Could you check a few things on this model? Use its own coordinates, in mm. A direction names the side the tool comes from. Round coordinates to 2 decimals unless told otherwise and drop trailing zeros. Loops run counter-clockwise (first coordinate to the right, second up) from the corner with the lowest first, then second, coordinate; pieces in that order, holes last. Notation, with made-up numbers: (35.5, -36.75) -> (77.5, -36.75) arc R36 cw to (77.5, -0.75) -> close; hole circle Ø6 at (47, 64). An arc over 180 degrees is marked (long way). One line per item, written item: value.
Autodesk Inventor part; units mm, degrees
ref_plane "YZ Plane" through (0, 0, 0) normal (1, 0, 0) x (0, 1, 0)
ref_plane "XZ Plane" through (0, 0, 0) normal (0, 1, 0) x (-1, 0, 0)
ref_plane "XY Plane" through (0, 0, 0) normal (0, 0, 1) x (1, 0, 0)
sketch "Boceto1" plane through (0, 0, 0) normal (0, 0, 1) x (1, 0, 0)
  point P0 (0, 0)
sketch "Boceto2" plane through (0, 0, 0) normal (0, 0, 1) x (1, 0, 0)
  line L0 (0, 0) -> (0, 200)
  line L1 (0, 200) -> (600, 200)
  line L2 (600, 200) -> (600, 0)
  line L3 (600, 0) -> (0, 0)
  dimension "d0" = 200
  dimension "d1" = 600
  dimension "d2" = 200
  dimension "d3" = 600
extrude "Extrusión1" add sketch "Boceto2" along normal blind 300
shell "Vaciado1" thickness 10 removed faces 1 at (400, 0, 100)
sketch "Boceto3" plane through (0, 200, 0) normal (0, 1, 0) x (1, 0, 0)
  point P0 (0, 0)
sketch "Boceto4" plane through (0, 200, 0) normal (0, 1, 0) x (1, 0, 0)
  point P0 (0, 0)
sketch "Boceto5" plane through (0, 200, 0) normal (0, 1, 0) x (1, 0, 0)
  point P0 (0, 0)
sketch "Boceto6" plane through (0, 200, 0) normal (0, 1, 0) x (1, 0, 0)
  circle A0 centre (300, -150) radius 15
  point P0 (0, 0)
  dimension "d9" = 30
extrude "Extrusión2" cut sketch "Boceto6" against normal blind 33.25
sketch "Boceto7" plane through (0, 200, 0) normal (0, 1, 0) x (1, 0, 0)
  point P0 (0, 0)
sketch "Boceto8" plane through (600, 0, 0) normal (1, 0, 0) x (0, 0, -1)
  circle A0 centre (-22.0681, 21.036) radius 17.5
  circle A1 centre (-69.9749, 21.036) radius 17.5
  point P0 (0, 0)
  dimension "d12" = 35
  dimension "d13" = 35
extrude "Extrusión3" cut sketch "Boceto8" against normal blind 33.25
sketch "Boceto9" plane through (0, 0, 0) normal (-1, 0, 0) x (0, 0, 1)
  arc A0 (10, 8.3628) -> (10, 33.7092) centre (22.0681, 21.036) ccw
  circle A1 centre (22.0681, 21.036) radius 17.5
  circle A2 centre (66.1324, 21.036) radius 17.5
  point P0 (0, 0)
  dimension "d16" = 35
  dimension "d17" = 35
extrude "Extrusión4" cut sketch "Boceto9" against normal blind 10
(1) For pin 1 Ø4 at (x, z) = (104, 207.5) entering from -Y, with a flat end and sliding along its axis, tell me the tip position at first contact or that it passes through.
Results below:
pin 1: stops at y = 190
(2) Imagine slicing it at A-A on z = 150. Write out the boundary of the cut face in (x, y), then the cut area to 3 significant figures.
Results below:
outline: (0, 0) -> (10, 0) -> (10, 190) -> (285, 190) -> (285, 200) -> (0, 200) -> close; (315, 190) -> (590, 190) -> (590, 0) -> (600, 0) -> (600, 200) -> (315, 200) -> close
area: 9,500 mm²
(3) On a 3-axis mill with a long thin cutter (end or side, diameter ignored), from which of +Z, -Z, +X, -X, +Y, -Y can I reach the whole of each face in a straight line? I mean faces 1 (the face through (296, 190, 179)), 2 (the face through (590.997, 26.293, 5.376)), 3 (the face through (600, 101, 148)), 4 (the face through (4.93, 14.333, 82.298)). Say none if no direction works.
Results below:
face 1: -Y
face 2: +X
face 3: +Z, -Z, +X, +Y, -Y
face 4: -X
(4) Imagine slicing it at B-B on x = 300. Write out the boundary of the cut face in (y, z).
Results below:
outline: (0, 0) -> (200, 0) -> (200, 135) -> (190, 135) -> (190, 10) -> (0, 10) -> close; (0, 290) -> (190, 290) -> (190, 165) -> (200, 165) -> (200, 300) -> (0, 300) -> close
(5) Please list where these lines run through material, in increasing order: L1, parallel to Z at x = 300, y = 194.5; L2, parallel to Z at x = 140, y = 129.5; L3, parallel to X at y = 195.25, z = 150.
Results below:
L1: z = 0 to 135, 165 to 300
L2: z = 0 to 10, 290 to 300
L3: x = 0 to 285, 315 to 600
(6) Imagine slicing it at D-D on z = 78. Write out the boundary of the cut face in (x, y), then the cut area to 3 significant figures.
Results below:
outline: (0, 0) -> (10, 0) -> (10, 8.17) -> (0, 8.17) -> close; (0, 33.9) -> (10, 33.9) -> (10, 190) -> (590, 190) -> (590, 36.59) -> (600, 36.59) -> (600, 200) -> (0, 200) -> close; (590, 0) -> (600, 0) -> (600, 5.48) -> (590, 5.48) -> close
area: 9,230 mm²
(7) Imagine slicing it at C-C on y = 128. Write out the boundary of the cut face in (x, z).
Results below:
outline: (0, 0) -> (600, 0) -> (600, 300) -> (0, 300) -> close; hole (10, 10) -> (590, 10) -> (590, 290) -> (10, 290) -> close
(8) We'd pull the mould along Y, two halves only. Please class faces 5 (the face through (296, 200, 181)), 6 (the face through (296, 96, 10)), 7 (the face through (4.93, 20.46, 39.56)), 8 (the face through (595.07, 21.805, 87.458)): +Y half, -Y half, draft (parallel to the pull), parting line (faces both ways), or undercut.
Results below:
face 5: +Y half
face 6: draft
face 7: undercut
face 8: undercut
